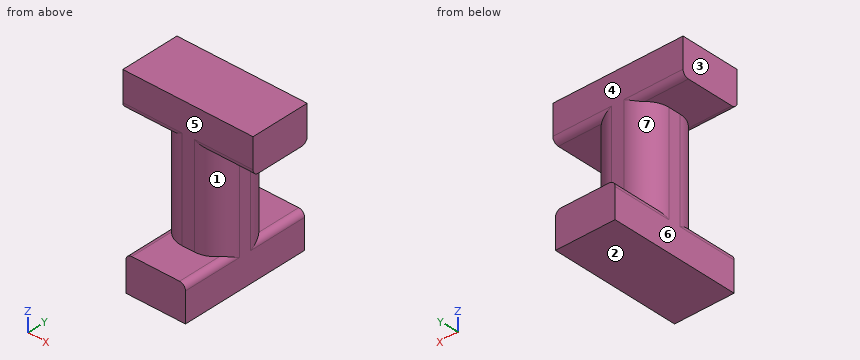
```python
from build123d import *

# Parameters (mm, degrees)
ESQUISSE1_W         = 5.035107038
ESQUISSE1_H         = 5
BASE_DEPTH          = 8
BOSS_1_DEPTH        = 3
BOSS_1_DEPTH_BACK   = 8
ESQUISSE4_W         = 5.035107038
ESQUISSE4_H         = 3
BOSS_2_DEPTH        = 3
BOSS_2_DEPTH_BACK   = 8
ESQUISSE5_W         = 3
ESQUISSE5_H         = 5
CONGE_MILIEU_R      = 2
CONGE_HAUT_ET_BAS_R = 0.5


with BuildPart() as part:
    # Esquisse1 → BASE (new body)
    with BuildSketch(Plane.XY):
        with Locations((34.295782161, 18.98164147)):
            Rectangle(ESQUISSE1_W, ESQUISSE1_H)
    extrude(amount=BASE_DEPTH)

    # Esquisse4 → BOSS 1 (add, two sides: drawn at the far end of the back side and taken through both)
    with BuildSketch(Plane(origin=(0, 21.48164147, 0), x_dir=(1, 0, 0), z_dir=(0, 1, 0)).offset(-BOSS_1_DEPTH_BACK)):
        with Locations((34.295782161, 1.5)):
            Rectangle(ESQUISSE4_W, ESQUISSE4_H)
    extrude(amount=BOSS_1_DEPTH + BOSS_1_DEPTH_BACK)

    # Esquisse5 → BOSS 2 (add, two sides: drawn at the far end of the back side and taken through both)
    with BuildSketch(Plane.ZY.offset(-31.778228642).offset(-BOSS_2_DEPTH_BACK)):
        with Locations((9.5, 18.98164147)):
            Rectangle(ESQUISSE5_W, ESQUISSE5_H)
    extrude(amount=BOSS_2_DEPTH + BOSS_2_DEPTH_BACK)

    # CONGE MILIEU
    conge_milieu_edges = [part.edges().sort_by_distance(p)[0] for p in [
        (36.81333568, 21.48164147, 4),
        (31.778228642, 21.48164147, 4),
        (31.778228642, 16.48164147, 4),
        (36.81333568, 16.48164147, 4),
    ]]
    fillet(conge_milieu_edges, radius=CONGE_MILIEU_R)

    # CONGE HAUT ET BAS
    conge_haut_et_bas_edges = [part.edges().sort_by_distance(p)[0] for p in [
        (36.81333568, 15.98164147, 0),
        (36.81333568, 21.98164147, 0),
        (31.778228642, 15.98164147, 0),
        (31.778228642, 21.98164147, 0),
        (37.295782161, 16.48164147, 8),
        (31.278228642, 16.48164147, 8),
        (37.295782161, 21.48164147, 8),
        (31.278228642, 21.48164147, 8),
    ]]
    fillet(conge_haut_et_bas_edges, radius=CONGE_HAUT_ET_BAS_R)


solid = part.part
```
The model under review builds one solid part; all positions refer to its coordinate system, in mm. Face numbers are marked on the shaded views. A direction names the side the tool comes from. Round coordinates to 2 decimals unless told otherwise and drop trailing zeros. Loops run counter-clockwise (first coordinate to the right, second up) from the corner with the lowest first, then second, coordinate; pieces in that order, holes last. Notation, with made-up numbers: M 11.25,33 L 37.25,33 A14 cw 37.25,43 Z; hole C 32.5,72.25 d2. An arc over 180 degrees is marked long. Put each result on its own line as item: value.
Q1. Consider section A-A, the plane z = 1.75. Give the boundary of the cut face in (x, y).
Result set:
outline: M 31.78,18.48 A2 ccw 33.78,16.48 L 34.81,16.48 A2 ccw 36.81,18.48 L 36.81,19.48 A2 ccw 34.81,21.48 L 33.78,21.48 A2 ccw 31.78,19.48 Z
Q2. Machinability: for the marked faces 4, 5, 6 and 7, which of the approach directions +Z, -Z, +X, -X, +Y, -Y give a long, thin tool a straight path to every point of the face, cutting with its end or side? Answer none if there is none.
Result set:
face 4: +Z, +X, -X, +Y
face 5: +Z, +X, -X, -Y
face 6: -Z, -X, +Y, -Y
face 7: -X, +Y
Q3. Mouldability with a two-part tool opening along Z and no side actions: class the marked faces 1, 2 and 3 as released by +Z, released by -Z, zero draft, split by the parting line, or undercut.
Result set:
face 1: undercut
face 2: released by -Z
face 3: zero draft
Q4. Consider section C-C, the plane x = 29.75. Give the boundary of the cut face in (y, z), then the cut area to 3 significant figures.
Result set:
outline: M 16.48,8.5 A0.5 ccw 16.98,8 L 20.98,8 A0.5 ccw 21.48,8.5 L 21.48,11 L 16.48,11 Z
area: 14.9 mm²
Q5. Consider section D-D, the plane x = 35.5. Give the boundary of the cut face in (y, z).
Result set:
outline: M 13.48,-3 L 24.48,-3 L 24.48,0 L 21.36,0 L 21.36,8.17 A0.5 ccw 21.48,8.5 L 21.48,11 L 16.48,11 L 16.48,8.5 A0.5 ccw 16.6,8.17 L 16.6,0 L 13.48,0 Z
Q6. For pin 1 (5 mm diameter, centred on x = 34, y = 15.5, fed in from +Z); pin 2 (3.5 mm diameter, centred on x = 36, z = 6.5, fed in from -Y); pin 3 (1.5 mm diameter, centred on x = 36, z = 1, fed in from +Y); pin 4 (2 mm diameter, centred on y = 16.5, z = 0, fed in from -X), all flat-tipped, find the tip position at first contact; note any pin that passes through.
Result set:
pin 1: stops at z = 11
pin 2: stops at y = 16.48
pin 3: stops at y = 21.43
pin 4: stops at x = 31.78
Q7. Consider section B-B, the plane y = 15.5. Give the boundary of the cut face in (x, z).
Result set:
outline: M 31.78,-3 L 36.81,-3 L 36.81,-0.5 A0.5 ccw 36.31,0 L 32.28,0 A0.5 ccw 31.78,-0.5 Z
Q8. To check wall thickness, follow L1, parallel to Z at x = 34.5, y = 23.25; L2, parallel to Y at x = 34.5, z = 1.5; L3, parallel to X at y = 21.5, z = -2. State the ranges of each line that lie inside material, in increasing order.
Result set:
L1: z = -3 to 0
L2: y = 16.48 to 21.48
L3: x = 31.78 to 36.81
